Autodesk Inventor part; units mm, degrees
ref_plane "YZ Plane" through (0, 0, 0) normal (1, 0, 0) x (0, 1, 0)
ref_plane "XZ Plane" through (0, 0, 0) normal (0, 1, 0) x (-1, 0, 0)
ref_plane "XY Plane" through (0, 0, 0) normal (0, 0, 1) x (1, 0, 0)
sketch "Эскиз1" plane through (0, 0, 0) normal (0, 0, 1) x (1, 0, 0)
  circle A0 centre (0, 0) radius 17.5
  circle A1 centre (0, 0) radius 25
  dimension "d0" = 35
  dimension "d1" = 50
extrude "Выдавливание1" add sketch "Эскиз1" along normal blind 10
sketch "Эскиз2" plane through (0, 0, 10) normal (0, 0, 1) x (1, 0, 0)
  circle A0 centre (0, 0) radius 17.5
  circle A1 centre (0, 0) radius 21
  dimension "d4" = 42
extrude "Выдавливание2" add sketch "Эскиз2" along normal blind 18
sketch "Эскиз5" plane through (0, 0, 28) normal (0, 0, 1) x (1, 0, 0)
  circle A0 centre (0, 0) radius 21
  circle A1 centre (0, 0) radius 17.5
  circle A2 centre (0, 0) radius 30
  dimension "d20" = 60
extrude "Выдавливание5" add sketch "Эскиз5" along normal blind 1 contours A0 | A2
sketch "Эскиз3" plane through (0, 0, 29) normal (0, 0, 1) x (1, 0, 0)
  circle A0 centre (0, 0) radius 21
  circle A1 centre (0, 0) radius 30
  circle A2 centre (0, 0) radius 25
  dimension "d7" = 60
  dimension "d13" = 50
extrude "Выдавливание3" add sketch "Эскиз3" along normal blind 50 contours A1
chamfer "Фаска1" distance 4 angle 45 1 edges at (-25, 0, 10)
sketch "Эскиз4" plane through (0, 0, 0) normal (0, 0, -1) x (-1, 0, 0)
  circle A0 centre (0, 0) radius 17.5
  circle A1 centre (0, 0) radius 20
  dimension "d17" = 40
extrude "Выдавливание4" add sketch "Эскиз4" along normal blind 8
chamfer "Фаска3" distance 9 angle 45 1 edges at (-21, 0, 28)
sketch "Эскиз6" plane through (0, 0, 79) normal (0, 0, 1) x (1, 0, 0)
  circle A0 centre (0, 0) radius 30
  circle A1 centre (0, 0) radius 25
  circle A2 centre (0, 0) radius 35
  dimension "d26" = 70
extrude "Выдавливание6" add sketch "Эскиз6" along normal blind 2 contours A0 | A2
sketch "Эскиз7" plane through (0, 0, 81) normal (0, 0, 1) x (1, 0, 0)
  circle A0 centre (0, 0) radius 35
  circle A1 centre (0, 0) radius 30
  dimension "d29" = 60
extrude "Выдавливание7" add sketch "Эскиз7" along normal blind 7
chamfer "Фаска4" distance 5 angle 45 1 edges at (-30, 0, 79)
sketch "Эскиз8" plane through (0, 0, 0) normal (0, 1, 0) x (-1, 0, 0)
  line L0 (30, 81) -> (-30, 81)
  line L1 (30, 81) -> (30, 83)
  line L2 (30, 88) -> (30, 81)
  line L3 (30, 83) -> (32, 83)
  line L4 (32, 83) -> (32, 85)
  line L5 (32, 85) -> (30, 85)
  line L6 (0, -27.2) -> (0, 107.2)
  point P0 (0, 0)
  dimension "d35" = 2
  dimension "d36" = 2
  dimension "d37" = 2
revolve "Вращение1" cut sketch "Эскиз8" angle 360 about axis through (0, 0, -10) along (0, 0, 1)
properties part number "Для регулировки 3" material "Сталь, высокопрочная, низколегированная"
Here's how the part is built. I have some questions about the finished solid (model axes, mm). A direction names the side the tool comes from. Coordinates: 2 decimals unless noted, no trailing zeros. Order: outer loops, then holes, each group sorted by start corner. A loop starts at its lowest first (then second) coordinate and runs counter-clockwise, first axis right, second up. Notation, with made-up numbers: (-26.75, 32) -> (-12.75, 32) arc R23 cw to (-12.75, 58) -> close; hole circle Ø1 at (-39.75, -23.5). An arc over 180 degrees is marked (long way). Answer in a Markdown table with one row per item.
(1) On a 3-axis mill with a long thin cutter (end or side, diameter ignored), from which of +Z, -Z, +X, -X, +Y, -Y can I reach the whole of each face in a straight line? I mean faces 1 (the face through (23.846, -7.509, 2.958)), 2 (the face through (-9, -29, 85)), 3 (the face through (-7, 25, 81)). Say none if no direction works.
Answer key:
| item | result |
|---|---|
| face 1 | -Z |
| face 2 | none |
| face 3 | +Z |
(2) I want a section at B-B on z = 14.5. List the corners of the cut face in (x, y) for me, then the cut area to 3 significant figures.
Answer key:
| item | result |
|---|---|
| outline | circle Ø42 at (0, 0); hole circle Ø35 at (0, 0) |
| area | 423 mm^2 |
(3) I want a section at A-A on z = 69. List the corners of the cut face in (x, y) for me.
Answer key:
| item | result |
|---|---|
| outline | circle Ø60 at (0, 0); hole circle Ø50 at (0, 0) |
(4) Will these pins go through, and if not, where does the flat tip stop? pin 1 Ø6 at (x, z) = (9.5, 18) entering from -Y; pin 2 Ø12.5 at (x, y) = (-10.5, -2.5) entering from +Z; pin 3 Ø1.5 at (y, z) = (2.5, 27) entering from -X; pin 4 Ø3 at (y, z) = (-19.5, 41) entering from -X.
Answer key:
| item | result |
|---|---|
| pin 1 | y = -21.19 |
| pin 2 | through |
| pin 3 | x = -29.65 |
| pin 4 | x = -24 |
(5) Please list where these lines run through material, in increasing order: probe 1 along Y at (x, z) = (0, 82); probe 2 along Y at (x, z) = (0, 69); probe 3 along X at (y, z) = (5, 30.5).
Answer key:
| item | result |
|---|---|
| probe 1 | -35 to -30, 30 to 35 |
| probe 2 | -30 to -25, 25 to 30 |
| probe 3 | -29.58 to -24.49, 24.49 to 29.58 |
(6) Thinking about a two-plate mould opening in Y: for faces 4 (the face through (-11, 17, 0)), 5 (the face through (-17, -5, 29)), 6 (the face through (-29.97, -1.32, 50.68)), 7 (the face through (6.94, 31.24, 84.01)), which applies, +Y half, -Y half, draft (parallel to the pull), parting line (faces both ways), or undercut?
Answer key:
| item | result |
|---|---|
| face 4 | draft |
| face 5 | undercut |
| face 6 | parting line |
| face 7 | undercut |
